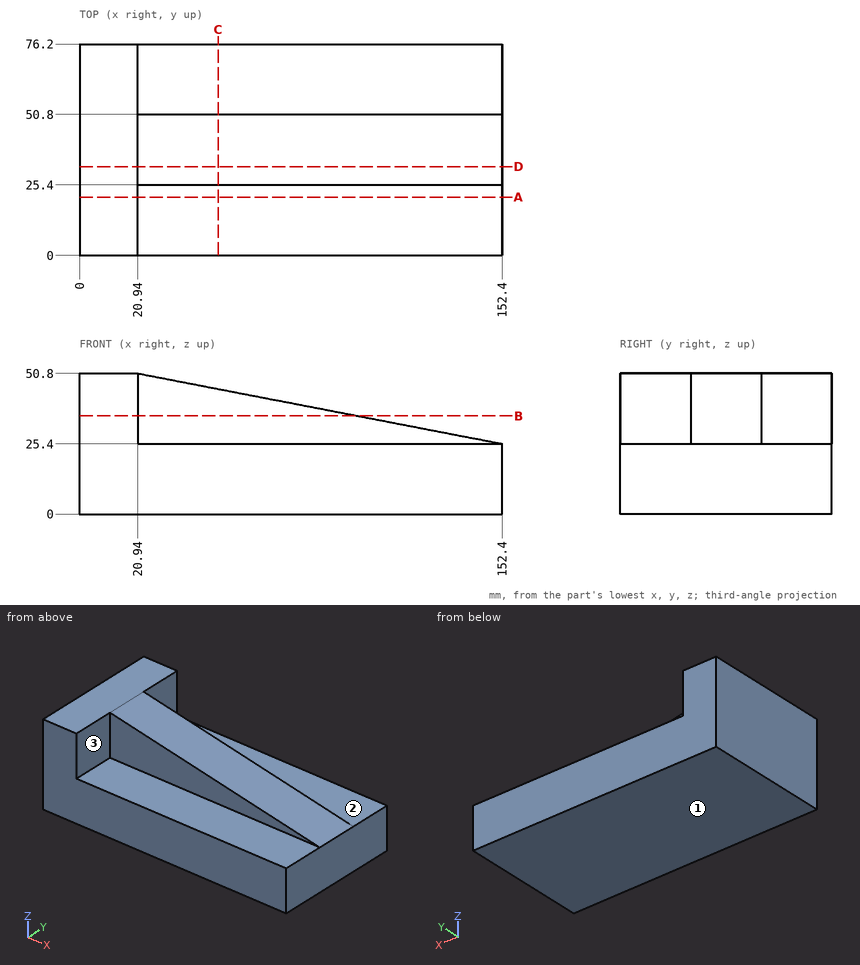
Study the drawing (mm; zero at the part's minimum x, y, z) and answer. A direction names the side the tool comes from. Coordinates: 2 decimals unless noted, no trailing zeros. Order: outer loops, then holes, each group sorted by start corner. A loop starts at its lowest first (then second) coordinate and runs counter-clockwise, first axis right, second up. Notation, with made-up numbers: (57.25, -21) -> (97.25, -21) arc R30 ccw to (97.25, 14) -> close; hole circle Ø3 at (-37, -35). An arc over 180 degrees is marked (long way). Answer in a Markdown table with one row per item. Add a question column.
Item 1: Find section A-A (y = 21). Write down the section's boundary in (x, z).
Item 2: Find the intervals of material crossed by L1, parallel to Z at x = 46, y = 70; L2, parallel to X at y = 60.5, z = 32.5; L3, parallel to Y at x = 117.5, z = 25.5, in increasing order. Write a range as from..to.
Item 3: Find section C-C (x = 50). Write down the section's boundary in (y, z) (3 decimals), then the cut area to 3 significant figures.
Item 4: Each of these flat-tipped pins is pushed along its axis until it touches: P1, Ø7.5, axis at y = 65, z = 33.5, coming from the +X side; P2, Ø5, axis at x = 132.5, y = 35.5, coming from the -Z side; P3, Ø20.5, axis at x = 62.5, y = 61.5, coming from the +Z side; P4, Ø10, axis at x = 28.5, y = 24.5, coming from the +Z side. Where does it stop, or does it pass through?
Item 5: Find section B-B (z = 35.5). Write down the section's boundary in (x, y).
Item 6: Which of the six approach directions +Z, -Z, +X, -X, +Y, -Y give full straight-line access (tool end or side, diameter ignored) to the marked faces 1, 2 and 3?
Item 7: Find section D-D (y = 32). Write down the section's boundary in (x, z).
Result set:
| question | item | result |
|---|---|---|
| 1 | outline | (0, 0) -> (152.4, 0) -> (152.4, 25.4) -> (20.94, 25.4) -> (20.94, 50.8) -> (0, 50.8) -> close |
| 2 | L1 | z = 0..25.4 |
| 2 | L2 | x = 0..20.94 |
| 2 | L3 | y = 25.4..50.8 |
| 3 | outline | (0, 0) -> (76.2, 0) -> (76.2, 25.4) -> (50.8, 25.4) -> (50.8, 45.185) -> (25.4, 45.185) -> (25.4, 25.4) -> (0, 25.4) -> close |
| 3 | area | 2,440 mm² |
| 4 | P1 | stops at x = 20.94 |
| 4 | P2 | stops at z = 0 |
| 4 | P3 | stops at z = 25.4 |
| 4 | P4 | stops at z = 50.29 |
| 5 | outline | (0, 0) -> (20.94, 0) -> (20.94, 25.4) -> (100.13, 25.4) -> (100.13, 50.8) -> (20.94, 50.8) -> (20.94, 76.2) -> (0, 76.2) -> close |
| 6 | face 1 | -Z, +X, -X, +Y, -Y |
| 6 | face 2 | +Z, +X, +Y |
| 6 | face 3 | +Z, +X, -Y |
| 7 | outline | (0, 0) -> (152.4, 0) -> (152.4, 25.4) -> (20.94, 50.8) -> (0, 50.8) -> close |
